Geometry check sheet. Reference: the model listing, model coordinates, mm. Coordinates: 2 decimals unless noted, no trailing zeros. Order: outer loops, then holes, each group sorted by start corner. A loop starts at its lowest first (then second) coordinate and runs counter-clockwise, first axis right, second up. Notation, with made-up numbers: M -39.5,45.25 L -23.5,45.25 A26 cw -23.5,72.25 Z; hole C 67,51.25 d7. An arc over 180 degrees is marked long. One line per item, written item: value. Start each with the question number.
1) Sectioned sample at A-A, the plane x = 0. Enter the section's corners in (y, z), then the cut area to 3 significant figures.
2) Go/stop test with a flat-tipped pin: P1, Ø1.4, axis at x = -19.6, z = 10.4, coming from the -Y side. Record where the tip stops, or that it passes through.
3) Thickness scan on L1, parallel to Z at x = 0, y = 0.3; L2, parallel to Z at x = -9, y = 0.25; L3, parallel to X at y = 0.25, z = -12. Record the ranges inside material, lowest first. Write a range as from..to.
4) Draft check along Z on faces 1 (the flat face through (0, 0.8, -5)), 2 (the cylindrical face through (-21.147, 0.394, 8.247)), 3 (the cylindrical face through (18.89, 0.406, 10.036)). Enter one of: pulls with the +Z half, pulls with the -Z half, needs draft (parallel to the pull), parting line crosses it, or undercut.
5) Sectioned sample at B-B, the plane z = 15. Enter the section's corners in (x, y), then the cut area to 3 significant figures.
```python
from build123d import *

# Parameters (mm, degrees)
BOSS_EXTRUDE1_DEPTH = 0.8
CUT_EXTRUDE1_DEPTH  = 1.8000001
SKETCH3_R           = 0.8
CUT_EXTRUDE2_DEPTH  = 1.8000001


with BuildPart() as part:
    # Sketch1 → Boss-Extrude1 (new body)
    with BuildSketch(Plane(origin=(0, 0, 0), x_dir=(1, 0, 0), z_dir=(0, 1, 0))):
        with BuildLine():
            Line((3.5, 32.496165092), (-3.5, 32.496165092))
            add(Edge.make_bspline(
                [(-3.5, 32.496165092), (-18.367827069, 28.850667185), (-21.698636831, 6.25)],
                knots=[3.299552084, 3.299552084, 3.299552084, 4.489304273, 4.489304273, 4.489304273], degree=2, weights=[1, 0.828217943, 1]))
            Line((-21.698636831, 6.25), (-21.698636831, -6.25))
            ThreePointArc((-21.698636831, -6.25), (-15.212563947, -17.564440685), (-3.5, -23.300428417))
            Line((-3.5, -23.300428417), (3.5, -23.300428417))
            ThreePointArc((3.5, -23.300428417), (15.212563947, -17.564440685), (21.698636831, -6.25))
            Line((21.698636831, -6.25), (21.698636831, 6.25))
            add(Edge.make_bspline(
                [(21.698636831, 6.25), (18.367827069, 28.850667185), (3.5, 32.496165092)],
                knots=[1.793881034, 1.793881034, 1.793881034, 2.983633223, 2.983633223, 2.983633223], degree=2, weights=[1, 0.828217943, 1]))
        make_face()
    extrude(amount=BOSS_EXTRUDE1_DEPTH)

    # Sketch2 → Cut-Extrude1 (cut, through all)
    with BuildSketch(Plane.XZ):
        with BuildLine():
            Line((-8.95, -20.772566383), (9.95, -20.772566383))
            ThreePointArc((9.95, -20.772566383), (10.45, -21.272566383), (9.95, -21.772566383))
            Line((9.95, -21.772566383), (-8.95, -21.772566383))
            ThreePointArc((-8.95, -21.772566383), (-9.45, -21.272566383), (-8.95, -20.772566383))
        make_face()
    extrude(amount=-CUT_EXTRUDE1_DEPTH, mode=Mode.SUBTRACT)

    # Sketch3 → Cut-Extrude2 (cut, through all)
    with BuildSketch(Plane(origin=(0, 0.8, 0), x_dir=(1, 0, 0), z_dir=(0, 1, 0))):
        with Locations((0, 32.272488183)):
            Circle(SKETCH3_R)
        with Locations((19.60344615, -10.397433617)):
            Circle(SKETCH3_R)
        with Locations((-19.60344615, -10.397433617)):
            Circle(SKETCH3_R)
    extrude(amount=-CUT_EXTRUDE2_DEPTH, mode=Mode.SUBTRACT)


solid = part.part
```
Final values:
1. outline: M 0,-31.47 L 0.8,-31.47 L 0.8,-21.77 L 0,-21.77 Z; M 0,-20.77 L 0.8,-20.77 L 0.8,23.3 L 0,23.3 Z
1. area: 43.0 mm^2
2. P1: passes through
3. L1: z = -31.47..-21.77, -20.77..23.3
3. L2: z = -30..-21.77, -20.78..21.68
3. L3: x = -20.5..20.5
4. face 1: needs draft
4. face 2: pulls with the +Z half
4. face 3: undercut
5. outline: M -17.55,0 L 17.55,0 L 17.55,0.8 L -17.55,0.8 Z
5. area: 28.1 mm^2
